Autodesk Inventor part; units mm, degrees
ref_plane "YZ Plane" through (0, 0, 0) normal (1, 0, 0) x (0, 1, 0)
ref_plane "XZ Plane" through (0, 0, 0) normal (0, 1, 0) x (-1, 0, 0)
ref_plane "XY Plane" through (0, 0, 0) normal (0, 0, 1) x (1, 0, 0)
sketch "Szkic1" plane through (0, 0, 0) normal (0, 1, 0) x (-1, 0, 0)
  line L0 (-35, 45) -> (35, 45)
  line L1 (40, 40) -> (40, -40)
  line L2 (35, -45) -> (-35, -45)
  line L3 (-40, -40) -> (-40, -25)
  line L4 (-40, 45) -> (40, -45) construction
  line L5 (40, 45) -> (-40, -45) construction
  arc A0 (40, 40) -> (35, 45) centre (35, 40) ccw
  arc A1 (-35, 45) -> (-40, 40) centre (-35, 40) ccw
  arc A2 (-40, -40) -> (-35, -45) centre (-35, -40) ccw
  arc A3 (35, -45) -> (40, -40) centre (35, -40) ccw
  line L6 (15, -25) -> (-5, -25)
  line L7 (-5, -25) -> (-5, 16)
  line L8 (-5, 16) -> (15, 16)
  line L9 (15, 16) -> (15, -25)
  circle A4 centre (10, 19.25) radius 2.5
  circle A5 centre (0, 19.25) radius 2.5
  circle A6 centre (10, -28.25) radius 2.5
  circle A7 centre (0, -28.25) radius 2.5
  line L10 (-40, 25) -> (-35, 25)
  line L11 (-35, 25) -> (-35, 20)
  line L12 (-35, 20) -> (-40, 20)
  line L13 (-40, -20) -> (-35, -20)
  line L14 (-35, -20) -> (-35, -25)
  line L15 (-35, -25) -> (-40, -25)
  line L16 (-40, 20) -> (-40, 25)
  line L17 (-40, 25) -> (-40, 40)
  line L18 (-40, -20) -> (-40, 20)
  circle A8 centre (-22, -35) radius 2.5
  circle A9 centre (-22, 35) radius 2.5
  circle A10 centre (-31, 35) radius 2.5
  circle A11 centre (-31, -35) radius 2.5
  point P0 (0, 0)
  dimension "d0" = 80
  dimension "d1" = 90
  dimension "d2" = 5
  dimension "d3" = 20
  dimension "d4" = 41
  dimension "d5" = 5
  dimension "d6" = 5
  dimension "d7" = 5
  dimension "d8" = 5
  dimension "d18" = 5
  dimension "d19" = 5
  dimension "d20" = 5
  dimension "d21" = 5
  dimension "d50" = 5
  dimension "d52" = 5
  dimension "d53" = 5
  dimension "d54" = 5
extrude "Wyciągnięcie proste3" add sketch "Szkic1" along normal blind 5 contours L0 A0 L1 A3 L2 A2 L3 L15 L14 L13 L18 L12 L11 L10 L17 A1
properties part number "Ground"
Check sheet for the modelled part. Datum: model origin and axes. Units: mm. A direction names the side the tool comes from. Coordinates: 2 decimals unless noted, no trailing zeros. Loops run counter-clockwise (first coordinate to the right, second up) from the corner with the lowest first, then second, coordinate; pieces in that order, holes last. Notation, with made-up numbers: (84, -11.75) -> (129, -11.75) arc R29 cw to (129, 14.25) -> close; hole circle Ø5 at (-9, -33). An arc over 180 degrees is marked (long way). Answer in a Markdown table with one row per item.
1. Material ranges on line 1 along X through (y, z) = (3.2, -28); line 2 along Z through (x, y) = (31, 1.4); line 3 along X through (y, z) = (1.3, 13), recorded low to high. Write a range as [from, to].
Check values:
| item | result |
|---|---|
| line 1 | x = [-40, -12.49], [-7.51, -2.49], [2.49, 40] |
| line 2 | z = [-45, -37.5], [-32.5, 32.5], [37.5, 45] |
| line 3 | x = [-40, -15], [5, 40] |
2. Release check for a two-part mould opening along Z. For faces 4 (the face through (24.5, 2.5, -35.1)), 5 (the face through (38, 2, -44)), 6 (the face through (-38, 2, 44)), 7 (the face through (-15, 2, -4)) record: released by +Z, released by -Z, zero draft, split by the parting line, or undercut.
Check values:
| item | result |
|---|---|
| face 4 | undercut |
| face 5 | released by -Z |
| face 6 | released by +Z |
| face 7 | undercut |
3. Sectioned sample at C-C, the plane y = 2.9. Give the number of separate pieces and of enclosed holes in the cut face, then the cut area to 3 significant figures.
Check values:
| item | result |
|---|---|
| separate pieces | 1 |
| enclosed holes | 9 |
| area | 6,150 mm2 |
4. Sectioned sample at D-D, the plane z = 13. Record the boundary of the cut face in (x, y).
Check values:
| item | result |
|---|---|
| outline | (-40, 0) -> (-15, 0) -> (-15, 5) -> (-40, 5) -> close; (5, 0) -> (40, 0) -> (40, 5) -> (5, 5) -> close |
5. Sectioned sample at A-A, the plane x = -10. Record the boundary of the cut face in (y, z).
Check values:
| item | result |
|---|---|
| outline | (0, -45) -> (5, -45) -> (5, -30.75) -> (0, -30.75) -> close; (0, -25.75) -> (5, -25.75) -> (5, -25) -> (0, -25) -> close; (0, 16) -> (5, 16) -> (5, 16.75) -> (0, 16.75) -> close; (0, 21.75) -> (5, 21.75) -> (5, 45) -> (0, 45) -> close |
6. Sectioned sample at B-B, the plane z = 35. Record the boundary of the cut face in (x, y).
Check values:
| item | result |
|---|---|
| outline | (-40, 0) -> (19.5, 0) -> (19.5, 5) -> (-40, 5) -> close; (24.5, 0) -> (28.5, 0) -> (28.5, 5) -> (24.5, 5) -> close; (33.5, 0) -> (40, 0) -> (40, 5) -> (33.5, 5) -> close |
7. Go/stop test with flat-tipped pins: pin 1 (2.5 mm diameter, centred on x = 38, y = 3, fed in from -Z); pin 2 (1.5 mm diameter, centred on y = 3, z = 23.5, fed in from +X); pin 3 (1.5 mm diameter, centred on x = 37, y = 2.5, fed in from -Z). Record where each tip stops, or that it passes through.
Check values:
| item | result |
|---|---|
| pin 1 | stops at z = -44.68 |
| pin 2 | stops at x = 35 |
| pin 3 | stops at z = -44.84 |
8. Access from +Z, -Z, +X, -X, +Y, -Y to the whole of each face (thin tool, end or side, straight path). Record for faces 1 (the face through (35, 2, 23)), 2 (the face through (-40, 2, 1)), 3 (the face through (5, 2, -5)).
Check values:
| item | result |
|---|---|
| face 1 | +X, +Y, -Y |
| face 2 | +Z, -Z, -X, +Y, -Y |
| face 3 | +Y, -Y |
